Build history of the part. All positions in model axes, mm. Face numbers are marked on the shaded views. A direction names the side the tool comes from. Give positions to 0.01 mm unless a question says otherwise; leave off trailing zeros. Write each loop counter-clockwise with the first axis right and the second up, starting at its lowest first coordinate (ties: lowest second). Pieces come first, ordered by that corner, then holes. Notation, with made-up numbers: M 84.25,39.5 L 117.25,39.5 A23 cw 117.25,52.5 Z; hole C 37.5,78 d1. An arc over 180 degrees is marked long. Return JSON: item names as keys, results as strings. Group by question number.
Q1. Tool access for the marked faces 4 and 5: list every direction of +Z, -Z, +X, -X, +Y, -Y with a clear straight run to the whole face (end or side of a thin tool).
Q2. Band-saw the part on C-C, the plane z = 342. Give the cut face in (x, y).
Q3. Flat gauge pins, fed straight in: pin 1 Ø5 at (y, z) = (-102, 219) entering from -X; pin 2 Ø5 at (y, z) = (-155.5, 125.5) entering from +X; pin 3 Ø6 at (y, z) = (-159, 72.5) entering from +X. Where does each tip first touch, or does it go through?
Q4. Pull direction X, two halves, no side cores. Call the marked faces 1, 2 and 3: +X half, -X half, draft (parallel to the pull), parting line (faces both ways), or undercut.
Q5. Band-saw the part on A-A, the plane x = -29. Give the cut face in (y, z), then the cut area to 3 significant figures.
Q6. Wall check: probe 1 along Z at (x, y) = (-76, -138); probe 2 along X at (y, z) = (-211.5, 181.5); probe 3 along X at (y, z) = (-118.5, 388). Give the ranges that are in metal, low to high.
Q7. Band-saw the part on B-B, the plane y = -139. Give the cut face in (x, z), then the cut area to 3 significant figures.
Q8. Band-saw the part on D-D, the plane x = 74.5. Give the cut face in (y, z).
from build123d import *

# Parameters (mm, degrees)
F1_DEPTH = 250
F3_DEPTH = 250.001
F4_W     = 200
F4_H     = 400
F5_DEPTH = 1.5


with BuildPart() as f1:
    # F0 (on Front) → F1 (new body)
    with BuildSketch(Plane.XZ):
        Polygon((-153.1775129723, 18), (-153.1775129723, 0), (226.53011856, 0), (36.3519007767, 407.8385041665), (-118.1775129723, 407.8385041665), (-118.1775129723, 18), align=None)
    extrude(amount=F1_DEPTH)

    # F2 (on face) → F3 (cut, through all)
    with BuildSketch(Plane(origin=(0, 0, 0), x_dir=(-1, 0, 0), z_dir=(0, 1, 0))):
        Polygon((-198.2757781719, 18), (100.1775129723, 18), (100.1775129723, 389.8385041665), (-24.8846360822, 389.8385041665), align=None)
    extrude(amount=-F3_DEPTH, mode=Mode.SUBTRACT)

    # F4 (on face) → F5 (join)
    with BuildSketch(Plane(origin=(186.0704359956, 0, 86.766069261), x_dir=(0, 1, 0), z_dir=(0.906307787, 0, 0.4226182617))):
        with Locations((-125, 129.2642350622)):
            Rectangle(F4_W, F4_H)
    extrude(amount=F5_DEPTH)


solid = f1.part
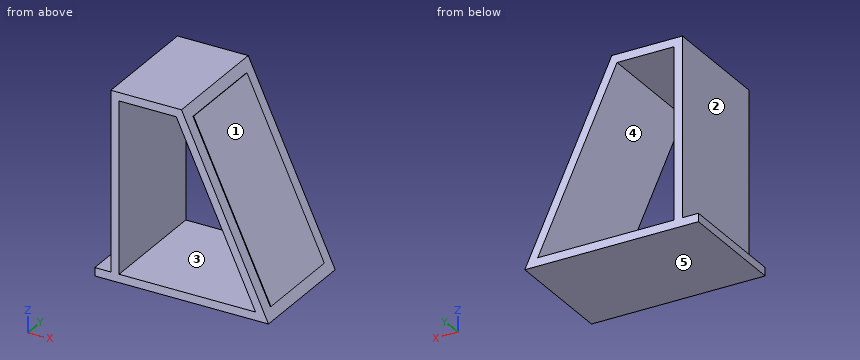
From the geometry:
{
 "1": {"face 4": "+Y, -Y", "face 5": "-Z, +X, -X, +Y, -Y"},
 "2": {"outline": "M -118.18,-250 L -100.18,-250 L -100.18,0 L -118.18,0 Z; M 47.19,-250 L 67.05,-250 L 67.05,-225 L 68.71,-225 L 68.71,-25 L 67.05,-25 L 67.05,0 L 47.19,0 Z"},
 "3": {"pin 1": "stops at x = -118.18", "pin 2": "stops at x = 170.83", "pin 3": "stops at x = 195.78"},
 "4": {"face 1": "+X half", "face 2": "-X half", "face 3": "undercut"},
 "5": {"outline": "M -250,0 L 0,0 L 0,18 L -250,18 Z; M -250,389.84 L 0,389.84 L 0,407.84 L -250,407.84 Z", "area": "9,000 mm^2"},
 "6": {"probe 1": "z = 0 to 18, 389.84 to 407.84", "probe 2": "x = -118.18 to -100.18, 122.03 to 143.55", "probe 3": "x = -118.18 to -100.18, 25.74 to 45.6"},
 "7": {"outline": "M -153.18,0 L 226.53,0 L 215.96,22.66 L 217.32,23.29 L 48.28,385.81 L 46.92,385.18 L 36.35,407.84 L -118.18,407.84 L -118.18,18 L -153.18,18 Z; hole M -100.18,18 L 198.28,18 L 24.88,389.84 L -100.18,389.84 Z", "area": "24,300 mm^2"},
 "8": {"outline": "M -250,0 L 0,0 L 0,18 L -250,18 Z; M -250,283.44 L 0,283.44 L 0,326.03 L -25,326.03 L -25,329.58 L -225,329.58 L -225,326.03 L -250,326.03 Z"}
}
